from build123d import *

# Parameters (mm, degrees)
F0_W     = 50.8
F0_H     = 5.08
F1_DEPTH = 38.1
F2_R     = 0.635
F3_DEPTH = 6.35


# Not quite as in the source:
# - a pattern or mirror of a feature is missing from the dataset's text; its kind, count and spacing are read off the source's solid


with BuildPart() as f1:
    # F0 (on Front) → F1 (new body, symmetric)
    with BuildSketch(Plane.XZ):
        Rectangle(F0_W, F0_H)
    extrude(amount=F1_DEPTH, both=True)

    # F2 (on face) → F3 (cut)
    with BuildSketch(Plane.XZ.offset(38.1)):
        with Locations((-19.05, 1.27)):
            Circle(F2_R)
        with BuildLine():
            ThreePointArc((-13.335, 1.27), (-13.1490128061, 0.8209871939), (-12.7, 0.635))
            Line((-12.7, 0.635), (0, 0.635))
            Line((0, 0.635), (12.7, 0.635))
            ThreePointArc((12.7, 0.635), (13.1490128061, 0.8209871939), (13.335, 1.27))
            Line((13.335, 1.27), (13.335, 2.54))
            Line((13.335, 2.54), (-13.335, 2.54))
            Line((-13.335, 2.54), (-13.335, 1.27))
        make_face()
        with Locations((19.05, 1.27)):
            Circle(F2_R)
    f3 = extrude(amount=-F3_DEPTH, mode=Mode.SUBTRACT)

    # F3_copies: F3 across plane
    add(f3.mirror(Plane.ZX), mode=Mode.SUBTRACT)


solid = f1.part
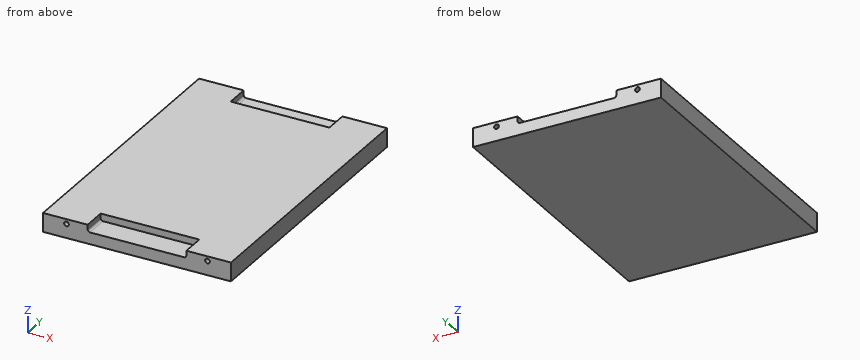
Model file for the job. Use its own axes, mm. Coordinates: 2 decimals unless noted, no trailing zeros. Write each loop counter-clockwise with the first axis right and the second up, starting at its lowest first coordinate (ties: lowest second). Pieces come first, ordered by that corner, then holes. Notation, with made-up numbers: (88.25, -9.75) - (147.25, -9.75) arc R10 ccw to (147.25, 4.25) - close; hole circle Ø3 at (49, 37). An arc over 180 degrees is marked (long way). Write each question's results on one line, items separated by ' | '. Start each with the question number.
1) Cut at B-B (x = -9). Write the cut outline in (y, z) (3 decimals).
2) Flat gauge pins, fed straight in: P1, Ø1.1, axis at x = -19.05, z = 1.27, coming from the -Y side; P2, Ø1, axis at x = 2, z = 1.5, coming from the +Y side; P3, Ø3, axis at x = 4.5, y = -34, coming from the +Z side (3 decimals). Where does each tip first touch, or does it go through?
3) Probe line 1 along Z through (x, y) = (-19, -35); line 2 along Y through (x, z) = (-3, 1.8). List the from-to ranges inside material, lowest first. Write a range as from..to.
4) Cut at A-A (y = -32.5). Write the cut outline in (x, z) (3 decimals).
Returned:
1) outline: (-38.1, -2.54) - (38.1, -2.54) - (38.1, 0.635) - (31.75, 0.635) - (31.75, 2.54) - (-31.75, 2.54) - (-31.75, 0.635) - (-38.1, 0.635) - close
2) P1: y = -31.75 | P2: y = 31.75 | P3: z = 0.635
3) line 1: -2.54..0.64, 1.9..2.54 | line 2: -31.75..31.75
4) outline: (-25.4, -2.54) - (25.4, -2.54) - (25.4, 2.54) - (13.335, 2.54) - (13.335, 1.27) arc R0.635 cw to (12.7, 0.635) - (-12.7, 0.635) arc R0.635 cw to (-13.335, 1.27) - (-13.335, 2.54) - (-25.4, 2.54) - close; hole circle Ø1.27 at (-19.05, 1.27); hole circle Ø1.27 at (19.05, 1.27)
